Could you check a few things on this model? Use its own coordinates, in mm. Face numbers are marked on the shaded views. Give positions to 0.01 mm unless a question says otherwise; leave off trailing zeros. Order: outer loops, then holes, each group sorted by start corner. A loop starts at its lowest first (then second) coordinate and runs counter-clockwise, first axis right, second up. Notation, with made-up numbers: M 34.25,-29.75 L 69.25,-29.75 A33 cw 69.25,3.25 Z; hole C 14.5,87 d1. An arc over 180 degrees is marked long. Return JSON: item names as keys, results as strings. Group by question number.
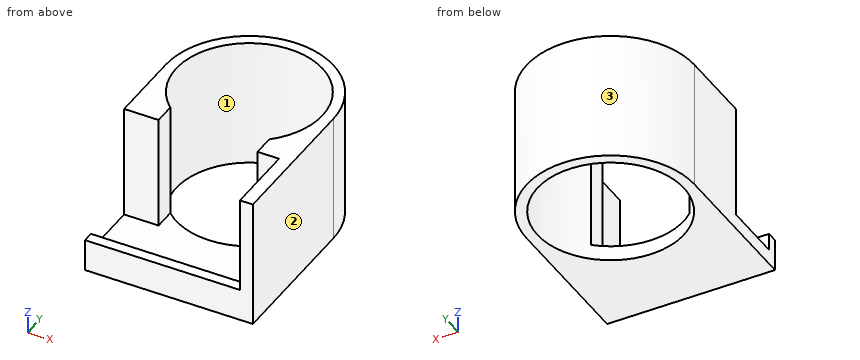
```python
from build123d import *

# Parameters (mm, degrees)
SKETCH1_R               = 49.53
SKETCH1_R_2             = 43.18
BOSS_EXTRUDE1_DEPTH     = 76.2
BOSS_EXTRUDE2_DEPTH     = 76.2
CUT_EXTRUDE4_DEPTH      = 91.44
CUT_EXTRUDE5_DEPTH      = 20.066
CUT_EXTRUDE5_DEPTH_BACK = 23.622


with BuildPart() as part:
    # Sketch1 → Boss-Extrude1 (new body)
    with BuildSketch(Plane.XY):
        Circle(SKETCH1_R)
        Circle(SKETCH1_R_2, mode=Mode.SUBTRACT)
    extrude(amount=BOSS_EXTRUDE1_DEPTH)

    # Sketch2 → Boss-Extrude2 (add)
    with BuildSketch(Plane.XY):
        with BuildLine():
            ThreePointArc((49.53, 0), (0, -49.53), (-49.53, 0))
            Line((-49.53, 0), (-49.53, -49.53))
            Line((-49.53, -49.53), (-49.53, -86.36))
            Line((-49.53, -86.36), (0, -86.36))
            Line((0, -86.36), (49.53, -86.36))
            Line((49.53, -86.36), (49.53, 0))
        make_face()
    extrude(amount=BOSS_EXTRUDE2_DEPTH)

    # Sketch3 → Cut-Extrude4 (cut)
    with BuildSketch(Plane.ZY.offset(49.53)):
        Polygon((19.065134697, -80.01), (19.065134697, -86.36), (31.768891325, -86.36), (76.2, -86.36), (76.2, -44.356391486), (8.879845192, -44.356391486), (8.879845192, -80.01), align=None)
    extrude(amount=-CUT_EXTRUDE4_DEPTH, mode=Mode.SUBTRACT)

    # Sketch6 → Cut-Extrude5 (cut, two sides)
    with BuildSketch(Plane.XZ.offset(44.356391486)) as cut_extrude5_sk:
        Polygon((0, 76.2), (-29.21, 76.2), (-29.21, 8.879845192), (29.21, 8.879845192), (29.21, 76.2), align=None)
    extrude(amount=CUT_EXTRUDE5_DEPTH, mode=Mode.SUBTRACT)
    extrude(cut_extrude5_sk.sketch, amount=-CUT_EXTRUDE5_DEPTH_BACK, mode=Mode.SUBTRACT)


solid = part.part
```
1. Imagine slicing it at D-D, the plane y = -73.5. Please give me the cut outline in (x, z).
2. Imagine slicing it at B-B, the plane y = 30. Please give me the cut outline in (x, z).
3. If we mould it in two halves opening along X, with no side actions, what happens to the marked faces 1, 2 and 3? For each: pulls with the +X half, pulls with the -X half, needs draft (parallel to the pull), parting line crosses it, or undercut.
4. Imagine slicing it at A-A, the plane x = 0. Please give me the cut outline in (y, z).
5. For pin 1 (3 mm diameter, centred on x = 1.5, y = -82, fed in from +Z); pin 2 (1.5 mm diameter, centred on x = -28, z = 58.5, fed in from +Y); pin 3 (5 mm diameter, centred on x = 12, y = -48.5, fed in from +Z), each with a flat end and sliding along its axis, tell me the tip position at first contact or that it passes through.
6. I need wall thicknesses on L1, parallel to X at y = 0, z = 57; L2, parallel to Y at x = 0, z = 24; L3, parallel to Z at x = 4, y = -45. Which ranges of each line are inside material? Lowest first, please. Write a range as from..to.
7. Imagine slicing it at C-C, the plane z = 7. Please give me the cut outline in (x, y), plus the area to 3 significant figures.
Values:
{
 "1": {"outline": "M -49.53,0 L 49.53,0 L 49.53,76.2 L 41.91,76.2 L 41.91,8.88 L -49.53,8.88 Z"},
 "2": {"outline": "M -39.41,0 L -31.06,0 L -31.06,76.2 L -39.41,76.2 Z; M 31.06,0 L 39.41,0 L 39.41,76.2 L 31.06,76.2 Z"},
 "3": {"face 1": "undercut", "face 2": "pulls with the +X half", "face 3": "parting line crosses it"},
 "4": {"outline": "M -86.36,0 L -43.18,0 L -43.18,8.88 L -80.01,8.88 L -80.01,19.07 L -86.36,19.07 Z; M 43.18,0 L 49.53,0 L 49.53,76.2 L 43.18,76.2 Z"},
 "5": {"pin 1": "stops at z = 19.07", "pin 2": "stops at y = 41.36", "pin 3": "stops at z = 8.88"},
 "6": {"L1": "x = -49.53..-43.18, 43.18..49.53", "L2": "y = 43.18..49.53", "L3": "z = 0..8.88"},
 "7": {"outline": "M -49.53,-86.36 L 49.53,-86.36 L 49.53,0 A49.53 ccw -49.53,0 Z; hole C 0,0 d86.36", "area": "6,550 mm²"}
}
